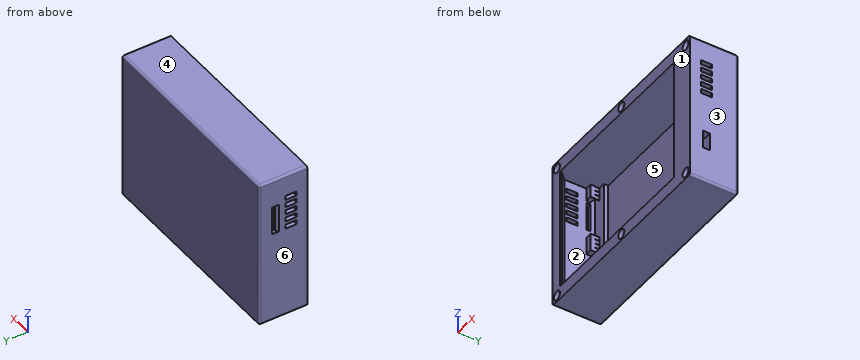
```python
from build123d import *

# Parameters (mm, degrees)
SKETCH_1_W               = 95
SKETCH_1_H               = 68
EXTRUDE_1_DEPTH          = 2
EXTRUDE_2_DEPTH          = 2
EXTRUDE_3_DEPTH          = 2
EXTRUDE_4_DEPTH          = 2
EXTRUDE_5_DEPTH          = 14
SKETCH_7_W               = 6
SKETCH_7_H               = 2
EXTRUDE_6_DEPTH          = 3
SKETCH_8_W               = 3
SKETCH_8_H               = 2
EXTRUDE_7_DEPTH          = 4
SKETCH_9_W               = 0.2
SKETCH_9_H               = 1.8
EXTRUDE_8_DEPTH          = 2
SKETCH_13_W              = 3
SKETCH_13_H              = 56
EXTRUDE_10_DEPTH         = 4
CHAMFER_6_SIZE           = 3
EXTRUDE_11_DEPTH         = 2
SKETCH_15_W              = 3
SKETCH_15_H              = 2
EXTRUDE_12_DEPTH         = 3
SKETCH_16_W              = 1.8
SKETCH_16_H              = 0.2
SKETCH_16_W_2            = 1
EXTRUDE_13_DEPTH         = 2
SKETCH_17_W              = 8
SKETCH_17_H              = 56
EXTRUDE_15_DEPTH         = 11
SKETCH_18_W              = 8
SKETCH_18_H              = 38
SKETCH_18_H_2            = 9.8
EXTRUDE_16_DEPTH         = 3.2
SKETCH_19_W              = 8
SKETCH_19_H              = 56
EXTRUDE_17_DEPTH         = 5.8
SKETCH_20_W              = 3
SKETCH_20_H              = 56
EXTRUDE_18_DEPTH         = 4
CHAMFER_7_SIZE           = 3
CHAMFER_8_SIZE           = 1
SKETCH_22_R              = 2.1
CUT_EXTRUDE_1_DEPTH      = 2.6
CUT_EXTRUDE_2_DEPTH      = 103.863987867
CUT_EXTRUDE_2_DEPTH_BACK = 103.863987867
SKETCH_23_W              = 2
SKETCH_23_H              = 5
FILLET_1_R               = 1
FILLET_2_R               = 1


with BuildPart() as part:
    # 草图1 → 凸台-拉伸1 (new body)
    with BuildSketch(Plane(origin=(0, 0, 0), x_dir=(1, 0, 0), z_dir=(0, 1, 0))):
        Rectangle(SKETCH_1_W, SKETCH_1_H)
    extrude(amount=EXTRUDE_1_DEPTH)

    # 草图3 → 凸台-拉伸2 (add)
    with BuildSketch(Plane.XZ):
        Polygon((-47.5, 34), (-39.5, 34), (47.5, 34), (47.5, 28), (-39.5, 28), (-39.5, -28), (47.5, -28), (47.5, -34), (-39.5, -34), (-47.5, -34), align=None)
    extrude(amount=EXTRUDE_2_DEPTH)

    # 草图4 → 凸台-拉伸3 (add)
    with BuildSketch(Plane.XZ.offset(2)):
        Polygon((-47.5, 34), (47.5, 34), (47.5, 28), (-45.5, 28), (-45.5, -28), (47.5, -28), (47.5, -34), (-47.5, -34), (-47.5, -28), (-47.5, 28), align=None)
    extrude(amount=EXTRUDE_3_DEPTH)

    # 草图5 → 凸台-拉伸4 (add)
    with BuildSketch(Plane.XZ.offset(4)):
        Polygon((-47.5, 34), (-45.5, 34), (47.5, 34), (47.5, 28), (-45.5, 28), (-45.5, 21), (-47.5, 21), align=None)
        Polygon((-47.5, 8), (-45.5, 8), (-45.5, -28), (47.5, -28), (47.5, -34), (-45.5, -34), (-47.5, -34), align=None)
    extrude(amount=EXTRUDE_4_DEPTH)

    # 草图6 → 凸台-拉伸5 (add)
    with BuildSketch(Plane.XZ.offset(6)):
        Polygon((-47.5, 34), (-45.5, 34), (47.5, 34), (47.5, 28), (-45.5, 28), (-45.5, -28), (47.5, -28), (47.5, -34), (-45.5, -34), (-47.5, -34), align=None)
    extrude(amount=EXTRUDE_5_DEPTH)

    # 草图7 → 凸台-拉伸6 (add)
    with BuildSketch(Plane(origin=(-45.5, 0, 0), x_dir=(0, 0, -1), z_dir=(1, 0, 0))):
        with Locations((-25, -5)):
            Rectangle(SKETCH_7_W, SKETCH_7_H)
        with Locations((-1, -5)):
            Rectangle(SKETCH_7_W, SKETCH_7_H)
    extrude(amount=EXTRUDE_6_DEPTH)

    # 草图8 → 凸台-拉伸7 (add)
    with BuildSketch(Plane.XZ.offset(2)):
        with Locations((-44, -3)):
            Rectangle(SKETCH_8_W, SKETCH_8_H)
    extrude(amount=EXTRUDE_7_DEPTH)

    # 草图9 → 凸台-拉伸8 (add)
    with BuildSketch(Plane.XZ.offset(2)):
        with Locations((-42.6, 22.9)):
            Rectangle(SKETCH_9_W, SKETCH_9_H)
        with Locations((-42.6, 24.9)):
            Rectangle(SKETCH_9_W, SKETCH_9_H)
        with Locations((-42.6, 26.9)):
            Rectangle(SKETCH_9_W, SKETCH_9_H)
        with Locations((-42.6, 3.1)):
            Rectangle(SKETCH_9_W, SKETCH_9_H)
        with Locations((-42.6, 1.1)):
            Rectangle(SKETCH_9_W, SKETCH_9_H)
        with Locations((-42.6, -0.9)):
            Rectangle(SKETCH_9_W, SKETCH_9_H)
    extrude(amount=EXTRUDE_8_DEPTH)

    # 草图13 → 凸台-拉伸10 (add)
    with BuildSketch(Plane.XZ.offset(20)):
        with Locations((-44, 0)):
            Rectangle(SKETCH_13_W, SKETCH_13_H)
    extrude(amount=-EXTRUDE_10_DEPTH)

    # 倒角6
    chamfer_6_edges = [part.edges().sort_by_distance(p)[0] for p in [
        (-42.5, -16, 0),
    ]]
    chamfer(chamfer_6_edges, length=CHAMFER_6_SIZE - 0.0001)  # a hair under: the kernel refuses the full size

    # 草图14 → 凸台-拉伸11 (add)
    with BuildSketch(Plane.XZ):
        Polygon((16.5, 28), (16.5, -2), (19.5, -2), (22.5, -2), (22.5, 28), (19.5, 28), align=None)
    extrude(amount=EXTRUDE_11_DEPTH)

    # 草图15 → 凸台-拉伸12 (add)
    with BuildSketch(Plane(origin=(0, 0, 28), x_dir=(-1, 0, 0), z_dir=(0, 0, -1))):
        with Locations((-18, -5)):
            Rectangle(SKETCH_15_W, SKETCH_15_H)
    extrude(amount=EXTRUDE_12_DEPTH)

    # 草图16 → 凸台-拉伸13 (add)
    with BuildSketch(Plane.XZ.offset(2)):
        with Locations((17.4, 25.1)):
            Rectangle(SKETCH_16_W, SKETCH_16_H)
        with Locations((19, 25.1)):
            Rectangle(SKETCH_16_W_2, SKETCH_16_H)
    extrude(amount=EXTRUDE_13_DEPTH)

    # 草图17 → 凸台-拉伸15 (add)
    with BuildSketch(Plane.XZ):
        with Locations((43.5, 0)):
            Rectangle(SKETCH_17_W, SKETCH_17_H)
    extrude(amount=EXTRUDE_15_DEPTH)

    # 草图18 → 凸台-拉伸16 (add)
    with BuildSketch(Plane.XZ.offset(11)):
        with Locations((43.5, 9)):
            Rectangle(SKETCH_18_W, SKETCH_18_H)
        with Locations((43.5, -23.1)):
            Rectangle(SKETCH_18_W, SKETCH_18_H_2)
    extrude(amount=EXTRUDE_16_DEPTH)

    # 草图19 → 凸台-拉伸17 (add)
    with BuildSketch(Plane.XZ.offset(14.2)):
        with Locations((43.5, 0)):
            Rectangle(SKETCH_19_W, SKETCH_19_H)
    extrude(amount=EXTRUDE_17_DEPTH)

    # 草图20 → 凸台-拉伸18 (add)
    with BuildSketch(Plane.XZ.offset(20)):
        with Locations((38, 0)):
            Rectangle(SKETCH_20_W, SKETCH_20_H)
    extrude(amount=-EXTRUDE_18_DEPTH)

    # 倒角7
    chamfer_7_edges = [part.edges().sort_by_distance(p)[0] for p in [
        (36.5, -16, 0),
    ]]
    chamfer(chamfer_7_edges, length=CHAMFER_7_SIZE - 0.0001)  # a hair under: the kernel refuses the full size

    # 倒角8
    chamfer_8_edges = [part.edges().sort_by_distance(p)[0] for p in [
        (-47.5, -6, 14.5),
    ]]
    chamfer(chamfer_8_edges, length=CHAMFER_8_SIZE)

    # 草图22 → 切除-拉伸1 (cut)
    with BuildSketch(Plane.XZ.offset(20)):
        with Locations(Location((-44.5, 31, 0), (0, 0, 270))):
            Circle(SKETCH_22_R)
        with Locations(Location((0, 31, 0), (0, 0, 270))):
            Circle(SKETCH_22_R)
        with Locations(Location((44.5, 31, 0), (0, 0, 270))):
            Circle(SKETCH_22_R)
        with Locations(Location((44.5, -31, 0), (0, 0, 270))):
            Circle(SKETCH_22_R)
        with Locations(Location((0, -31, 0), (0, 0, 270))):
            Circle(SKETCH_22_R)
        with Locations(Location((-44.5, -31, 0), (0, 0, 270))):
            Circle(SKETCH_22_R)
    extrude(amount=-CUT_EXTRUDE_1_DEPTH, mode=Mode.SUBTRACT)

    # 草图23 → 切除-拉伸2 (cut, two sides: drawn at the far end of the back side and taken through both)
    with BuildSketch(Plane(origin=(47.5, 0, 0), x_dir=(0, 0, -1), z_dir=(1, 0, 0)).offset(-CUT_EXTRUDE_2_DEPTH_BACK)):
        with Locations((-23, -12.5)):
            Rectangle(SKETCH_23_W, SKETCH_23_H)
        with Locations((-19.5, -12.5)):
            Rectangle(SKETCH_23_W, SKETCH_23_H)
        with Locations((-16, -12.5)):
            Rectangle(SKETCH_23_W, SKETCH_23_H)
        with Locations((-12.5, -12.5)):
            Rectangle(SKETCH_23_W, SKETCH_23_H)
        with Locations((-9, -12.5)):
            Rectangle(SKETCH_23_W, SKETCH_23_H)
    extrude(amount=CUT_EXTRUDE_2_DEPTH + CUT_EXTRUDE_2_DEPTH_BACK, mode=Mode.SUBTRACT)

    # 圆角1
    fillet_1_edges = [part.edges().sort_by_distance(p)[0] for p in [
        (-47.5, -9, -34),
        (47.5, -9, -34),
        (47.5, -9, 34),
        (-47.5, -9, 34),
    ]]
    fillet(fillet_1_edges, radius=FILLET_1_R)

    # 圆角2
    fillet_2_edges = [part.edges().sort_by_distance(p)[0] for p in [
        (0, 2, -34),
        (47.5, 2, 0),
        (-47.5, 2, 0),
        (0, 2, 34),
        (-47.207106781, 2, 33.707106781),
        (-47.207106781, 2, -33.707106781),
        (47.207106781, 2, 33.707106781),
        (47.207106781, 2, -33.707106781),
    ]]
    fillet(fillet_2_edges, radius=FILLET_2_R)


solid = part.part
```
Part model, mm, in its own coordinate system. Face numbers are marked on the shaded views. A direction names the side the tool comes from. Give positions to 0.01 mm unless a question says otherwise; leave off trailing zeros. Write each loop counter-clockwise with the first axis right and the second up, starting at its lowest first coordinate (ties: lowest second). Pieces come first, ordered by that corner, then holes. Notation, with made-up numbers: M 6,-19 L 22,-19 A9 cw 22,-12 Z; hole C 35.5,-10 d2. An arc over 180 degrees is marked long. Use CSV: the item, a comma, the result in double quotes.
Item 1: Slice it at B-B on x = 0. Write the cut outline in (y, z), plus the area to 3 significant figures.
Taken from the geometry:
outline,"M -20,-34 L 1,-34 A1 ccw 2,-33 L 2,33 A1 ccw 1,34 L -20,34 L -20,33.1 L -17.4,33.1 L -17.4,28.9 L -20,28.9 L -20,28 L 0,28 L 0,-28 L -20,-28 L -20,-28.9 L -17.4,-28.9 L -17.4,-33.1 L -20,-33.1 Z"
area,"354 mm²"
Item 2: Pull direction X, two halves, no side cores. Call the marked faces 3, 4, 5 and 6: +X half, -X half, draft (parallel to the pull), parting line (faces both ways), or undercut.
Taken from the geometry:
face 3,"+X half"
face 4,"draft"
face 5,"undercut"
face 6,"-X half"
Item 3: Pin check, flat tips, straight feed: P1, Ø1.3, axis at x = 43.5, z = -32, coming from the -Y side; P2, Ø3, axis at x = 19.5, z = -2, coming from the -Y side. Stop position of each tip, or through.
Taken from the geometry:
P1,"stops at y = -17.4"
P2,"stops at y = -2"
Item 4: Drill centre lines: probe 1 along X at (y, z) = (-18.2, -31); probe 2 along X at (y, z) = (-6.5, -21.5); probe 3 along Z at (x, y) = (-33, -3.75). Where is each one in solid material? Low to high.
Taken from the geometry:
probe 1,"x = -47.5 to -46.6, -42.4 to -2.1, 2.1 to 42.4, 46.6 to 47.5"
probe 2,"x = -47.5 to -45.5, 39.5 to 47.5"
probe 3,"z = -34 to -28, 28 to 34"
Item 5: Slice it at C-C on z = 9. State how many separate pieces and enclosed holes the cut face has, plus the area to 3 significant figures.
Taken from the geometry:
separate pieces,"4"
enclosed holes,"0"
area,"374 mm²"
Item 6: Slice it at D-D on z = 31. Write the cut outline in (x, y), plus the area to 3 significant figures.
Taken from the geometry:
outline,"M -47.5,-20 L -46.6,-20 L -46.6,-17.4 L -42.4,-17.4 L -42.4,-20 L -2.1,-20 L -2.1,-17.4 L 2.1,-17.4 L 2.1,-20 L 42.4,-20 L 42.4,-17.4 L 46.6,-17.4 L 46.6,-20 L 47.5,-20 L 47.5,1 A1 ccw 46.5,2 L -46.5,2 A1 ccw -47.5,1 Z"
area,"2,060 mm²"
Item 7: Which spindle directions (+Z, -Z, +X, -X, +Y, -Y) get a long thin tool onto all of the face, cutting with end or side? Do the marked faces 1 and 2. Say none if no direction does.
Taken from the geometry:
face 1,"+Z, -Z, +X, -X, -Y"
face 2,"none"
Item 8: Slice it at A-A on y = -8.5. Write the cut outline in (x, z), plus the area to 3 significant figures.
Taken from the geometry:
outline,"M -47.5,-33 A1 ccw -46.5,-34 L 46.5,-34 A1 ccw 47.5,-33 L 47.5,33 A1 ccw 46.5,34 L -46.5,34 A1 ccw -47.5,33 Z; hole M -45.5,-28 L 39.5,-28 L 39.5,28 L -45.5,28 Z"
area,"1,700 mm²"
